Build history of the part. All positions in model axes, mm. A direction names the side the tool comes from. Coordinates: 2 decimals unless noted, no trailing zeros. Order: outer loops, then holes, each group sorted by start corner. A loop starts at its lowest first (then second) coordinate and runs counter-clockwise, first axis right, second up. Notation, with made-up numbers: (59.25, 20.25) -> (109.25, 20.25) arc R8 cw to (109.25, 26.25) -> close; hole circle Ø2 at (60, 71.25). An arc over 180 degrees is marked (long way). Write each question's results on one line, items separated by ' | '.
from build123d import *

# Parameters (mm, degrees)
F1_DEPTH = 85
F2_R     = 15
F3_R     = 2


# Not quite as in the source:
# - a feature of the source that left no trace in its solid (it failed there, or was rolled back) is left out


with BuildPart() as f1:
    # F0 (on Right) → F1 (new body)
    with BuildSketch(Plane.YZ):
        with BuildLine():
            Line((0, 4), (0, 0))
            Line((0, 0), (150, 0))
            Line((150, 0), (150, 4))
            Line((150, 4), (148.7324850447, 4))
            ThreePointArc((148.7324850447, 4), (147.4229901607, 4.4883045449), (146.7529275801, 5.7147768512))
            Line((146.7529275801, 5.7147768512), (142.6774710417, 34))
            Line((142.6774710417, 34), (138.7183561126, 33.4295537023))
            Line((138.7183561126, 33.4295537023), (140.5295339709, 11.9928994727))
            ThreePointArc((140.5295339709, 11.9928994727), (140.064889591, 10.5343894965), (138.7050141045, 9.8316203937))
            Line((138.7050141045, 9.8316203937), (120.5865966006, 8.3007995736))
            ThreePointArc((120.5865966006, 8.3007995736), (119.1280866244, 8.7654439535), (118.4253175217, 10.12531944))
            Line((118.4253175217, 10.12531944), (114.7183561126, 54))
            Line((114.7183561126, 54), (110.7183561126, 54))
            Line((110.7183561126, 54), (100.473891609, 16.4240136891))
            ThreePointArc((100.473891609, 16.4240136891), (98.862490978, 13.9077784109), (96.1038236872, 12.759820769))
            Line((96.1038236872, 12.759820769), (0, 4))
        make_face()
    extrude(amount=F1_DEPTH)

    # F2
    f2_edges = [f1.edges().sort_by_distance(p)[0] for p in [
        (85, 0, 2),
        (0, 0, 2),
    ]]
    fillet(f2_edges, radius=F2_R)

    # F3
    f3_edges = [f1.edges().sort_by_distance(p)[0] for p in [
        (42.5, 110.718356, 54),
        (42.5, 114.718356, 54),
        (42.5, 138.718356, 33.429554),
        (42.5, 142.677471, 34),
    ]]
    fillet(f3_edges, radius=F3_R)


solid = f1.part
Item 1: Slice it at B-B, the plane y = 47. List the corners of the cut face in (x, z), and give its area (3 significant figures).
Answer:
outline: (0, 0) -> (85, 0) -> (85, 8.28) -> (0, 8.28) -> close | area: 704 mm^2
Item 2: Tool access for faces 4 (the flat face through (42, 150, 2)), 5 (the flat face through (41.905, 129.773, 9.077)), 6 (the flat face through (41.9, 139.69, 21.91)): list every direction of +Z, -Z, +X, -X, +Y, -Y with a clear straight run to the whole face (end or side of a thin tool).
Answer:
face 4: +Z, -Z, +X, -X, +Y | face 5: +Z, +X, -X | face 6: +X, -X
Item 3: Drill centre lines: line 1 (Z direction, x = 7, y = 96); line 2 (Y direction, x = 10, z = 14); line 3 (Y direction, x = 60.5, z = 30). Where is each one in solid material? Low to high. Write a range as from..to.
Answer:
line 1: z = 0..12.75 | line 2: y = 98.97..118.1, 140.36..145.56 | line 3: y = 104.18..116.75, 139.01..143.25
Item 4: Slice it at A-A, the plane x = 66. List the corners of the cut face in (y, z), and give its area (3 significant figures).
Answer:
outline: (0, 0) -> (150, 0) -> (150, 4) -> (148.73, 4) arc R2 cw to (146.75, 5.71) -> (142.96, 32.02) arc R2 ccw to (140.7, 33.71) -> (140.58, 33.7) arc R2 ccw to (138.88, 31.55) -> (140.53, 11.99) arc R2 cw to (138.71, 9.83) -> (120.59, 8.3) arc R2 cw to (118.43, 10.13) -> (114.87, 52.17) arc R2 ccw to (112.88, 54) -> (112.25, 54) arc R2 ccw to (110.32, 52.53) -> (100.47, 16.42) arc R5 cw to (96.1, 12.76) -> (0, 4) -> close | area: 1,950 mm^2
Item 5: Slice it at C-C, the plane z = 49. List the corners of the cut face in (x, y).
Answer:
outline: (0, 109.36) -> (85, 109.36) -> (85, 115.14) -> (0, 115.14) -> close
Item 6: Pull direction Y, two halves, no side cores. Call faces 1 (the flat face through (0, 97, 11)), 2 (the flat face through (41.905, 116.674, 30.853)), 3 (the cylindrical face through (41.905, 98.895, 13.935)): released by +Y, released by -Y, zero draft, split by the parting line, or undercut.
Answer:
face 1: zero draft | face 2: undercut | face 3: released by -Y
Item 7: Pin check, flat tips, straight feed: pin 1 (5 mm diameter, centred on x = 42.5, z = 7.5, fed in from +Y); pin 2 (6 mm diameter, centred on x = 35, y = 39.5, fed in from +Z); pin 3 (1 mm diameter, centred on x = 26, y = 149.5, fed in from +Z). Stop position of each tip, or through.
Answer:
pin 1: stops at y = 147 | pin 2: stops at z = 7.87 | pin 3: stops at z = 4
